Geometry: final body of the model. Coordinates: model frame, mm. A direction names the side the tool comes from. Coordinates: 2 decimals unless noted, no trailing zeros. Write each loop counter-clockwise with the first axis right and the second up, starting at its lowest first coordinate (ties: lowest second). Pieces come first, ordered by that corner, then holes. Notation, with made-up numbers: (-23.5, 30) - (18.5, 30) arc R24 ccw to (18.5, 45) - close; hole circle Ø10 at (18.25, 7.25). An arc over 180 degrees is marked (long way). Answer as a JSON object with one key per item and string values. Group by question number.
Item 1: Set-up query: faces 1 (the flat face through (-77.696, 18, 2)), 2 (the flat face through (-79.196, 17.8, 0.4)), 3 (the cylindrical face through (-86.722, 12.448, 3.538)). Return all of +Z, -Z, +X, -X, +Y, -Y with unobstructed straight access to the full face (end or side cutting, diameter ignored); none if empty.
Item 2: Section A-A on y = 20.75. Return loops of the section in (x, z), and give its area (3 significant figures).
Item 3: First-contact query: pin 1 Ø3 at (x, y) = (-78.5, 21.5) entering from -Z; pin 2 Ø5 at (x, y) = (-63.5, 16) entering from +Z; pin 3 Ø2 at (x, z) = (-58.5, 2.5) entering from -Y; pin 4 Ø0.7 at (y, z) = (20, 0.5) entering from -X. Flat tips, straight axial feed; report the tip coordinate or a pass-through.
Item 4: Line query: line 1 along X through (y, z) = (13, 0.7); line 2 along Z through (x, y) = (-66.5, 14.25); line 3 along Z through (x, y) = (-91, 19). Output: solid intervals per line, ascending. Write a range as from..to.
Item 5: Section B-B on z = 4. Return loops of the section in (x, y), and give its area (3 significant figures).
Item 6: Section C-C on x = -77. Return loops of the section in (y, z).
Item 7: Section D-D on y = 24.25. Return loops of the section in (x, z).
```python
from build123d import *

# Parameters (mm, degrees)
CROQUIS1_W              = 25
CROQUIS1_H              = 15
SALIENTE_EXTRUIR1_DEPTH = 1.4
SALIENTE_EXTRUIR2_DEPTH = 15
REDONDEO1_R             = 2
CORTAR_EXTRUIR1_START   = -2.177124
CORTAR_EXTRUIR1_DEPTH   = 2.177124


with BuildPart() as part:
    # Croquis1 → Saliente-Extruir1 (new body)
    with BuildSketch(Plane.XY):
        with Locations((-66.695768458, 17.882653061)):
            Rectangle(CROQUIS1_W, CROQUIS1_H)
    extrude(amount=SALIENTE_EXTRUIR1_DEPTH)

    # Croquis3 → Saliente-Extruir2 (add)
    with BuildSketch(Plane.XZ.offset(-10.382653061)):
        Polygon((-79.195768458, 1.4), (-79.195768458, 2.9), (-94.195768458, 2.9), (-94.195768458, 4.4), (-77.695768458, 4.4), (-77.695768458, 1.4), align=None)
    extrude(amount=-SALIENTE_EXTRUIR2_DEPTH)

    # Redondeo1
    redondeo1_edges = [part.edges().sort_by_distance(p)[0] for p in [
        (-79.195768458, 17.882653061, 2.9),
        (-77.695768458, 17.882653061, 4.4),
    ]]
    fillet(redondeo1_edges, radius=REDONDEO1_R)

    # Croquis4 → Cortar-Extruir1 (cut)
    with BuildSketch(Plane.XY.offset(4.4).offset(CORTAR_EXTRUIR1_START)):
        with BuildLine():
            Line((-79.695768458, 25.382653061), (-94.195768458, 25.382653061))
            Line((-94.195768458, 25.382653061), (-94.195768458, 22.382653061))
            ThreePointArc((-94.195768458, 22.382653061), (-86.824341518, 23.295756187), (-79.695768458, 25.382653061))
        make_face()
        with BuildLine():
            Line((-94.195768458, 13.382653061), (-94.195768458, 10.382653061))
            Line((-94.195768458, 10.382653061), (-79.695768458, 10.382653061))
            ThreePointArc((-79.695768458, 10.382653061), (-86.824341518, 12.469549935), (-94.195768458, 13.382653061))
        make_face()
    extrude(amount=CORTAR_EXTRUIR1_DEPTH, mode=Mode.SUBTRACT)


solid = part.part
```
Checks:
{
 "1": {"face 1": "+Z, +X, +Y, -Y", "face 2": "-Z, -X, +Y, -Y", "face 3": "+Z, -Z, -X, -Y"},
 "2": {"outline": "(-94.2, 2.9) - (-81.2, 2.9) arc R2 cw to (-79.2, 0.9) - (-79.2, 0) - (-54.2, 0) - (-54.2, 1.4) - (-77.7, 1.4) - (-77.7, 2.4) arc R2 ccw to (-79.7, 4.4) - (-94.2, 4.4) - close", "area": "62.0 mm^2"},
 "3": {"pin 1": "z = 0", "pin 2": "z = 1.4", "pin 3": "through", "pin 4": "x = -79.2"},
 "4": {"line 1": "-79.2..-54.2", "line 2": "0..1.4", "line 3": "2.9..4.4"},
 "5": {"outline": "(-94.2, 13.38) arc R46.03 cw to (-79.7, 10.38) - (-78.5, 10.38) - (-78.5, 25.38) - (-79.7, 25.38) arc R46.03 cw to (-94.2, 22.38) - close", "area": "180 mm^2"},
 "6": {"outline": "(10.38, 0) - (25.38, 0) - (25.38, 1.4) - (10.38, 1.4) - close"},
 "7": {"outline": "(-83.03, 2.9) - (-81.2, 2.9) arc R2 cw to (-79.2, 0.9) - (-79.2, 0) - (-54.2, 0) - (-54.2, 1.4) - (-77.7, 1.4) - (-77.7, 2.4) arc R2 ccw to (-79.7, 4.4) - (-83.03, 4.4) - close"}
}
